from build123d import *

# Parameters (mm, degrees)
BOSS_EXTRUDE1_DEPTH = 15
SKETCH2_R           = 5
CUT_EXTRUDE2_DEPTH  = 30


with BuildPart() as part:
    # Sketch1 → Boss-Extrude1 (new, symmetric)
    with BuildSketch(Plane(origin=(0, 0, 0), x_dir=(0, 0, -1), z_dir=(1, 0, 0))):
        with BuildLine():
            Line((2.346516976, 14.815325109), (2.861072583, 12.168165995))
            ThreePointArc((2.861072583, 12.168165995), (2.918067048, 12.154624005), (2.974997424, 12.14081506))
            Line((2.974997424, 12.14081506), (4.635254916, 14.265847744))
            Line((4.635254916, 14.265847744), (4.729368569, 11.570785321))
            ThreePointArc((4.729368569, 11.570785321), (4.783542905, 11.548494156), (4.837612178, 11.52594935))
            Line((4.837612178, 11.52594935), (6.809857496, 13.365097863))
            Line((6.809857496, 13.365097863), (6.481211806, 10.688493511))
            ThreePointArc((6.481211806, 10.688493511), (6.531232059, 10.658002054), (6.581108865, 10.627276514))
            Line((6.581108865, 10.627276514), (8.816778784, 12.135254916))
            Line((8.816778784, 12.135254916), (8.073466098, 9.543015517))
            ThreePointArc((8.073466098, 9.543015517), (8.118100604, 9.50507457), (8.16255681, 9.466924861))
            Line((8.16255681, 9.466924861), (10.606601718, 10.606601718))
            Line((10.606601718, 10.606601718), (9.466924861, 8.16255681))
            ThreePointArc((9.466924861, 8.16255681), (9.50507457, 8.118100604), (9.543015517, 8.073466098))
            Line((9.543015517, 8.073466098), (12.135254916, 8.816778784))
            Line((12.135254916, 8.816778784), (10.627276514, 6.581108865))
            ThreePointArc((10.627276514, 6.581108865), (10.658002054, 6.531232059), (10.688493511, 6.481211806))
            Line((10.688493511, 6.481211806), (13.365097863, 6.809857496))
            Line((13.365097863, 6.809857496), (11.52594935, 4.837612178))
            ThreePointArc((11.52594935, 4.837612178), (11.548494156, 4.783542905), (11.570785321, 4.729368569))
            Line((11.570785321, 4.729368569), (14.265847744, 4.635254916))
            Line((14.265847744, 4.635254916), (12.14081506, 2.974997424))
            ThreePointArc((12.14081506, 2.974997424), (12.154624005, 2.918067048), (12.168165995, 2.861072583))
            Line((12.168165995, 2.861072583), (14.815325109, 2.346516976))
            Line((14.815325109, 2.346516976), (12.456733611, 1.03912836))
            ThreePointArc((12.456733611, 1.03912836), (12.461466672, 0.980738697), (12.465926038, 0.922327493))
            Line((12.465926038, 0.922327493), (15, 0))
            Line((15, 0), (12.465926038, -0.922327493))
            ThreePointArc((12.465926038, -0.922327493), (12.461466672, -0.980738697), (12.456733611, -1.03912836))
            Line((12.456733611, -1.03912836), (14.815325109, -2.346516976))
            Line((14.815325109, -2.346516976), (12.168165995, -2.861072583))
            ThreePointArc((12.168165995, -2.861072583), (12.154624005, -2.918067048), (12.14081506, -2.974997424))
            Line((12.14081506, -2.974997424), (14.265847744, -4.635254916))
            Line((14.265847744, -4.635254916), (11.570785321, -4.729368569))
            ThreePointArc((11.570785321, -4.729368569), (11.548494156, -4.783542905), (11.52594935, -4.837612178))
            Line((11.52594935, -4.837612178), (13.365097863, -6.809857496))
            Line((13.365097863, -6.809857496), (10.688493511, -6.481211806))
            ThreePointArc((10.688493511, -6.481211806), (10.658002054, -6.531232059), (10.627276514, -6.581108865))
            Line((10.627276514, -6.581108865), (12.135254916, -8.816778784))
            Line((12.135254916, -8.816778784), (9.543015517, -8.073466098))
            ThreePointArc((9.543015517, -8.073466098), (9.50507457, -8.118100604), (9.466924861, -8.16255681))
            Line((9.466924861, -8.16255681), (10.606601718, -10.606601718))
            Line((10.606601718, -10.606601718), (8.16255681, -9.466924861))
            ThreePointArc((8.16255681, -9.466924861), (8.118100604, -9.50507457), (8.073466098, -9.543015517))
            Line((8.073466098, -9.543015517), (8.816778784, -12.135254916))
            Line((8.816778784, -12.135254916), (6.581108865, -10.627276514))
            ThreePointArc((6.581108865, -10.627276514), (6.531232059, -10.658002054), (6.481211806, -10.688493511))
            Line((6.481211806, -10.688493511), (6.809857496, -13.365097863))
            Line((6.809857496, -13.365097863), (4.837612178, -11.52594935))
            ThreePointArc((4.837612178, -11.52594935), (4.783542905, -11.548494156), (4.729368569, -11.570785321))
            Line((4.729368569, -11.570785321), (4.635254916, -14.265847744))
            Line((4.635254916, -14.265847744), (2.974997424, -12.14081506))
            ThreePointArc((2.974997424, -12.14081506), (2.918067048, -12.154624005), (2.861072583, -12.168165995))
            Line((2.861072583, -12.168165995), (2.346516976, -14.815325109))
            Line((2.346516976, -14.815325109), (1.03912836, -12.456733611))
            ThreePointArc((1.03912836, -12.456733611), (0.980738697, -12.461466672), (0.922327493, -12.465926038))
            Line((0.922327493, -12.465926038), (0, -15))
            Line((0, -15), (-0.922327493, -12.465926038))
            ThreePointArc((-0.922327493, -12.465926038), (-0.980738697, -12.461466672), (-1.03912836, -12.456733611))
            Line((-1.03912836, -12.456733611), (-2.346516976, -14.815325109))
            Line((-2.346516976, -14.815325109), (-2.861072583, -12.168165995))
            ThreePointArc((-2.861072583, -12.168165995), (-2.918067048, -12.154624005), (-2.974997424, -12.14081506))
            Line((-2.974997424, -12.14081506), (-4.635254916, -14.265847744))
            Line((-4.635254916, -14.265847744), (-4.729368569, -11.570785321))
            ThreePointArc((-4.729368569, -11.570785321), (-4.783542905, -11.548494156), (-4.837612178, -11.52594935))
            Line((-4.837612178, -11.52594935), (-6.809857496, -13.365097863))
            Line((-6.809857496, -13.365097863), (-6.481211806, -10.688493511))
            ThreePointArc((-6.481211806, -10.688493511), (-6.531232059, -10.658002054), (-6.581108865, -10.627276514))
            Line((-6.581108865, -10.627276514), (-8.816778784, -12.135254916))
            Line((-8.816778784, -12.135254916), (-8.073466098, -9.543015517))
            ThreePointArc((-8.073466098, -9.543015517), (-8.118100604, -9.50507457), (-8.16255681, -9.466924861))
            Line((-8.16255681, -9.466924861), (-10.606601718, -10.606601718))
            Line((-10.606601718, -10.606601718), (-9.466924861, -8.16255681))
            ThreePointArc((-9.466924861, -8.16255681), (-9.50507457, -8.118100604), (-9.543015517, -8.073466098))
            Line((-9.543015517, -8.073466098), (-12.135254916, -8.816778784))
            Line((-12.135254916, -8.816778784), (-10.627276514, -6.581108865))
            ThreePointArc((-10.627276514, -6.581108865), (-10.658002054, -6.531232059), (-10.688493511, -6.481211806))
            Line((-10.688493511, -6.481211806), (-13.365097863, -6.809857496))
            Line((-13.365097863, -6.809857496), (-11.52594935, -4.837612178))
            ThreePointArc((-11.52594935, -4.837612178), (-11.548494156, -4.783542905), (-11.570785321, -4.729368569))
            Line((-11.570785321, -4.729368569), (-14.265847744, -4.635254916))
            Line((-14.265847744, -4.635254916), (-12.14081506, -2.974997424))
            ThreePointArc((-12.14081506, -2.974997424), (-12.154624005, -2.918067048), (-12.168165995, -2.861072583))
            Line((-12.168165995, -2.861072583), (-14.815325109, -2.346516976))
            Line((-14.815325109, -2.346516976), (-12.456733611, -1.03912836))
            ThreePointArc((-12.456733611, -1.03912836), (-12.461466672, -0.980738697), (-12.465926038, -0.922327493))
            Line((-12.465926038, -0.922327493), (-15, 0))
            Line((-15, 0), (-12.465926038, 0.922327493))
            ThreePointArc((-12.465926038, 0.922327493), (-12.461466672, 0.980738697), (-12.456733611, 1.03912836))
            Line((-12.456733611, 1.03912836), (-14.815325109, 2.346516976))
            Line((-14.815325109, 2.346516976), (-12.168165995, 2.861072583))
            ThreePointArc((-12.168165995, 2.861072583), (-12.154624005, 2.918067048), (-12.14081506, 2.974997424))
            Line((-12.14081506, 2.974997424), (-14.265847744, 4.635254916))
            Line((-14.265847744, 4.635254916), (-11.570785321, 4.729368569))
            ThreePointArc((-11.570785321, 4.729368569), (-11.548494156, 4.783542905), (-11.52594935, 4.837612178))
            Line((-11.52594935, 4.837612178), (-13.365097863, 6.809857496))
            Line((-13.365097863, 6.809857496), (-10.688493511, 6.481211806))
            ThreePointArc((-10.688493511, 6.481211806), (-10.658002054, 6.531232059), (-10.627276514, 6.581108865))
            Line((-10.627276514, 6.581108865), (-12.135254916, 8.816778784))
            Line((-12.135254916, 8.816778784), (-9.543015517, 8.073466098))
            ThreePointArc((-9.543015517, 8.073466098), (-9.50507457, 8.118100604), (-9.466924861, 8.16255681))
            Line((-9.466924861, 8.16255681), (-10.606601718, 10.606601718))
            Line((-10.606601718, 10.606601718), (-8.16255681, 9.466924861))
            ThreePointArc((-8.16255681, 9.466924861), (-8.118100604, 9.50507457), (-8.073466098, 9.543015517))
            Line((-8.073466098, 9.543015517), (-8.816778784, 12.135254916))
            Line((-8.816778784, 12.135254916), (-6.581108865, 10.627276514))
            ThreePointArc((-6.581108865, 10.627276514), (-6.531232059, 10.658002054), (-6.481211806, 10.688493511))
            Line((-6.481211806, 10.688493511), (-6.809857496, 13.365097863))
            Line((-6.809857496, 13.365097863), (-4.837612178, 11.52594935))
            ThreePointArc((-4.837612178, 11.52594935), (-4.783542905, 11.548494156), (-4.729368569, 11.570785321))
            Line((-4.729368569, 11.570785321), (-4.635254916, 14.265847744))
            Line((-4.635254916, 14.265847744), (-2.974997424, 12.14081506))
            ThreePointArc((-2.974997424, 12.14081506), (-2.918067048, 12.154624005), (-2.861072583, 12.168165995))
            Line((-2.861072583, 12.168165995), (-2.346516976, 14.815325109))
            Line((-2.346516976, 14.815325109), (-1.03912836, 12.456733611))
            ThreePointArc((-1.03912836, 12.456733611), (-0.980738697, 12.461466672), (-0.922327493, 12.465926038))
            Line((-0.922327493, 12.465926038), (0, 15))
            Line((0, 15), (0.922327493, 12.465926038))
            ThreePointArc((0.922327493, 12.465926038), (0.980738697, 12.461466672), (1.03912836, 12.456733611))
            Line((1.03912836, 12.456733611), (2.346516976, 14.815325109))
        make_face()
    extrude(amount=BOSS_EXTRUDE1_DEPTH, both=True)

    # Sketch2 → Cut-Extrude2 (cut)
    with BuildSketch(Plane(origin=(15, 0, 0), x_dir=(0, 0, -1), z_dir=(1, 0, 0))):
        Circle(SKETCH2_R)
    extrude(amount=-CUT_EXTRUDE2_DEPTH, mode=Mode.SUBTRACT)


solid = part.part
Verification items for the finished model (mm, model axes). A direction names the side the tool comes from. Give positions to 0.01 mm unless a question says otherwise; leave off trailing zeros. Write each loop counter-clockwise with the first axis right and the second up, starting at its lowest first coordinate (ties: lowest second). Pieces come first, ordered by that corner, then holes. Notation, with made-up numbers: (46, 81.25) - (60, 81.25) arc R12 cw to (60, 100.25) - close; hole circle Ø8 at (-24.5, -7). An arc over 180 degrees is marked (long way). Answer as CSV lines item,"result". Start each with the question number.
1. Sectioned sample at A-A (z = -3.75). Record the boundary of the cut face in (x, y).
2. Depth check by flat-ended pin: pin 1 (1.5 mm diameter, centred on x = 4, z = -4.5, fed in from -Y); pin 2 (1.5 mm diameter, centred on x = 5, y = -3, fed in from +Z); pin 3 (3 mm diameter, centred on x = -6, y = -8, fed in from +Z). Enter the tip coordinate at first touch or a pass-through.
3. Set-up check for faces 1 (the face through (0.21, 0.468, -13.715)), 2 (the face through (0.21, -10.82, -8.44)), 3 (the face through (0.21, -12.46, -5.84)), 4 (the face through (0.21, 13.65, 1.7)): record each of +Z, -Z, +X, -X, +Y, -Y from which the full face is reachable in a straight line by a thin tool's end or side.
4. Sectioned sample at C-C (z = 5.5). Record the boundary of the cut face in (x, y).
5. Sectioned sample at B-B (y = 10). Record the boundary of the cut face in (x, z).
6. Thickness scan on line 1 (Y direction, x = 9.25, z = 10.5); line 2 (Y direction, x = 9.5, z = -11.75); line 3 (Y direction, x = 4, z = 11). Record the ranges inside material, lowest first.
7. Draft check along Z on faces 5 (the face through (0.21, 6.65, 12.05)), 6 (the face through (0.21, 13.715, 0.468)), 7 (the face through (0.21, 2.61, -13.47)). Enter one of: pulls with the +Z half, pulls with the -Z half, needs draft (parallel to the pull), parting line crosses it, or undercut.
Derived:
1,outline,"(-15, -13.13) - (15, -13.13) - (15, -3.31) - (-15, -3.31) - close; (-15, 3.31) - (15, 3.31) - (15, 13.13) - (-15, 13.13) - close"
2,pin 1,"y = -14.27"
2,pin 2,"z = 14.82"
2,pin 3,"z = 13.37"
3,face 1,"-Z, +X, -X"
3,face 2,"+X, -X"
3,face 3,"+X, -X, -Y"
3,face 4,"+X, -X, +Y"
4,outline,"(-15, -12.14) - (15, -12.14) - (15, 12.14) - (-15, 12.14) - close"
5,outline,"(-15, -10.32) - (15, -10.32) - (15, -9.31) - (-15, -9.31) - close; (-15, -8.2) - (15, -8.2) - (15, 8.2) - (-15, 8.2) - close; (-15, 9.31) - (15, 9.31) - (15, 10.32) - (-15, 10.32) - close"
6,line 1,"-10.56 to -10.38, -8.35 to 8.35, 10.38 to 10.56"
6,line 2,"-8.71 to -8.25, -6.61 to -5.08, -4.72 to 4.72, 5.08 to 6.61, 8.25 to 8.71"
6,line 3,"-8.49 to -7.13, -6.52 to 6.52, 7.13 to 8.49"
7,face 5,"undercut"
7,face 6,"undercut"
7,face 7,"pulls with the -Z half"
